```python
from build123d import *

# Parameters (mm, degrees)
SKETCH2_W           = 127
SKETCH2_H           = 127
BOSS_EXTRUDE1_DEPTH = 6.35
SKETCH6_R           = 2.5527
CUT_EXTRUDE3_DEPTH  = 9.525
CUT_EXTRUDE4_REACH  = 93.356
SKETCH7_R           = 7.62


with BuildPart() as part:
    # Sketch2 → Boss-Extrude1 (new body)
    with BuildSketch(Plane(origin=(0, 0, 0), x_dir=(1, 0, 0), z_dir=(0, 1, 0))):
        with Locations((-1.871480339, 0)):
            Rectangle(SKETCH2_W, SKETCH2_H)
    extrude(amount=BOSS_EXTRUDE1_DEPTH)

    # Sketch6 → Cut-Extrude3 (cut)
    with BuildSketch(Plane(origin=(0, 6.35, 0), x_dir=(1, 0, 0), z_dir=(0, 1, 0))):
        with Locations(Location((-52.671480339, 57.15, 0), (0, 0, 270))):
            Circle(SKETCH6_R)
        with Locations(Location((-52.671480339, -57.15, 0), (0, 0, 270))):
            Circle(SKETCH6_R)
        with Locations(Location((48.928519661, -57.15, 0), (0, 0, 270))):
            Circle(SKETCH6_R)
        with Locations(Location((48.928519661, 57.15, 0), (0, 0, 270))):
            Circle(SKETCH6_R)
    extrude(amount=-CUT_EXTRUDE3_DEPTH, mode=Mode.SUBTRACT)

    # Sketch7 → Cut-Extrude4 (cut, up to next)
    with BuildSketch(Plane(origin=(0, 6.35, 0), x_dir=(1, 0, 0), z_dir=(0, 1, 0)), mode=Mode.PRIVATE) as cut_extrude4_sk1:
        with Locations(Location((-39.971480339, 0, 0), (0, 0, 270))):
            Circle(SKETCH7_R)
    cut_extrude4_tool1 = extrude(cut_extrude4_sk1.sketch, amount=-CUT_EXTRUDE4_REACH, mode=Mode.PRIVATE) & part.part
    add(cut_extrude4_tool1.solids().sort_by_distance((-39.97148, 6.35, 0))[0], mode=Mode.SUBTRACT)


solid = part.part
```
Geometry check sheet. Reference: the model listing, model coordinates, mm. Coordinates: 2 decimals unless noted, no trailing zeros. Write each loop counter-clockwise with the first axis right and the second up, starting at its lowest first coordinate (ties: lowest second). Pieces come first, ordered by that corner, then holes. Notation, with made-up numbers: M 15.5,-19 L 48.5,-19 A17 ccw 48.5,14 Z; hole C 13,45.25 d8. An arc over 180 degrees is marked long. One line per item, written item: value. Start each with the question number.
(1) Sectioned sample at A-A, the plane z = 0. Enter the section's corners in (x, y).
(2) Sectioned sample at C-C, the plane y = 4. Enter the section's corners in (x, z), and give its area (3 significant figures).
(3) Release check for a two-part mould opening along X. For faces 1 (the face through (61.629, 3, 1)), 2 (the face through (49.695, 3.219, -54.715)), 3 (the face through (-3, 0, -1)), 4 (the face through (-65.371, 3, 1)) record: released by +X, released by -X, zero draft, split by the parting line, or undercut.
(4) Sectioned sample at B-B, the plane z = 57.15. Enter the section's corners in (x, y), and give its area (3 significant figures).
(5) Scan lines: line 1 along X through (y, z) = (2.5, 57.15); line 2 along X through (y, z) = (4.75, -56.5); line 3 along Z through (x, y) = (-55, 4). Record each from-to range of solid material in increasing order. Write a range as [from, to].
Filled sheet:
1. outline: M -65.37,0 L -47.59,0 L -47.59,6.35 L -65.37,6.35 Z; M -32.35,0 L 61.63,0 L 61.63,6.35 L -32.35,6.35 Z
2. outline: M -65.37,-63.5 L 61.63,-63.5 L 61.63,63.5 L -65.37,63.5 Z; hole C -52.67,-57.15 d5.11; hole C -52.67,57.15 d5.11; hole C -39.97,0 d15.24; hole C 48.93,-57.15 d5.11; hole C 48.93,57.15 d5.11
2. area: 15,900 mm²
3. face 1: released by +X
3. face 2: undercut
3. face 3: zero draft
3. face 4: released by -X
4. outline: M -65.37,0 L -55.22,0 L -55.22,6.35 L -65.37,6.35 Z; M -50.12,0 L 46.38,0 L 46.38,6.35 L -50.12,6.35 Z; M 51.48,0 L 61.63,0 L 61.63,6.35 L 51.48,6.35 Z
4. area: 742 mm²
5. line 1: [-65.37, -55.22], [-50.12, 46.38], [51.48, 61.63]
5. line 2: [-65.37, -55.14], [-50.2, 46.46], [51.4, 61.63]
5. line 3: [-63.5, -58.2], [-56.1, 56.1], [58.2, 63.5]
